from build123d import *

# Parameters (mm, degrees)
SALIENTE_EXTRUIR1_DEPTH      = 7.21
SALIENTE_EXTRUIR2_DEPTH      = 7.21
SALIENTE_EXTRUIR2_DEPTH_BACK = 7.21
CORTAR_EXTRUIR2_DEPTH        = 28.232395202
CORTAR_EXTRUIR2_DEPTH_BACK   = 28.232395202
SALIENTE_EXTRUIR3_START      = -5.2099999
SALIENTE_EXTRUIR3_DEPTH      = 10.4199998
SALIENTE_EXTRUIR3_START_2    = -7.470713012
SALIENTE_EXTRUIR3_2_DEPTH    = 14.941425924
SALIENTE_EXTRUIR3_START_3    = -23.035921246
SALIENTE_EXTRUIR3_3_DEPTH    = 24.035921246


with BuildPart() as part:
    # Croquis1 → Saliente-Extruir1 (new, symmetric)
    with BuildSketch(Plane.XY):
        with BuildLine():
            add(Edge.make_bspline(
                [(-18.945192114, 7.540918896), (-10.215008384, -3.697644103), (-2.846604825, -5.059081104)],
                knots=[0.497667241, 0.497667241, 0.497667241, 0.49955428, 0.49955428, 0.49955428], degree=2, weights=[1, 1, 1]))
            add(Edge.make_bspline(
                [(-2.846604825, -5.059081104), (-0.742366882, -3.9352066), (0.355125, -2.723253227)],
                knots=[0.498812075, 0.498812075, 0.498812075, 0.499412845, 0.499412845, 0.499412845], degree=2, weights=[1, 1, 1]))
            Line((0.355125, -2.723253227), (0.355125, -2.284841781))
            Line((0.355125, -2.284841781), (-1.394875, -2.223730435))
            add(Edge.make_bspline(
                [(-1.394875, -2.223730435), (-0.90753067, -0.123730435), (-1.394875, 1.976269565)],
                knots=[0, 0, 0, 1, 1, 1], degree=2, weights=[1, 3.231801219, 1]))
            Line((-1.394875, 1.976269565), (0.355125, 2.284841781))
            Line((0.355125, 2.284841781), (0.355125, 3.001549529))
            add(Edge.make_bspline(
                [(0.355125, 3.001549529), (-1.44872627, 6.058427314), (-6.994875026, 10.477389992)],
                knots=[0.500820705, 0.500820705, 0.500820705, 0.502013312, 0.502013312, 0.502013312], degree=2, weights=[1, 1, 1]))
            Line((-6.994875026, 10.477389992), (-8.981845695, 12.608155172))
            Line((-8.981845695, 12.608155172), (-23.035921146, 11.871612288))
            Line((-23.035921146, 11.871612288), (-23.035921146, 11.54013782))
            ThreePointArc((-23.035921146, 11.54013782), (-20.949684518, 9.582335705), (-18.945192114, 7.540918896))
        make_face()
    extrude(amount=SALIENTE_EXTRUIR1_DEPTH, both=True)

    # Croquis4 → Saliente-Extruir2 (add, two sides: drawn at the far end of the back side and taken through both)
    with BuildSketch(Plane.XY.offset(-SALIENTE_EXTRUIR2_DEPTH_BACK)):
        Polygon((-1.394875, 1.976269565), (0.355125, 2.284841781), (0.355125, 1.976269565), align=None)
    extrude(amount=SALIENTE_EXTRUIR2_DEPTH + SALIENTE_EXTRUIR2_DEPTH_BACK)

    # Croquis6 → Cortar-Extruir2 (cut, two sides: drawn at the far end of the back side and taken through both)
    with BuildSketch(Plane(origin=(0, 0, 0), x_dir=(0, 0, -1), z_dir=(1, 0, 0)).offset(-CORTAR_EXTRUIR2_DEPTH_BACK)):
        Polygon((7.21, 12.608155172), (7.21, -5.059081104), (5.21, -5.059081104), align=None)
        Polygon((-7.21, 12.608155172), (-7.21, -5.059081104), (-5.21, -5.059081104), align=None)
    extrude(amount=CORTAR_EXTRUIR2_DEPTH + CORTAR_EXTRUIR2_DEPTH_BACK, mode=Mode.SUBTRACT)

    # Saliente-Extruir3: read off the stored shape, not the designer's step
    # Saliente-Extruir3 outline → Saliente-Extruir3 (add)
    with BuildSketch(Plane.XY.offset(SALIENTE_EXTRUIR3_START)):
        with BuildLine():
            add(Edge.make_bspline(
                [(-9.626736117, 12.574357897), (-9.652391468, 12.594799115), (-9.678046818, 12.615240333)],
                knots=[0.502296281, 0.502296281, 0.502296281, 0.502301797, 0.502301797, 0.502301797], degree=2))
            Line((-9.626736117, 12.574357897), (-8.981845695, 12.608155172))
            Line((-8.981845695, 12.608155172), (-6.994875026, 10.477389992))
            add(Edge.make_bspline(
                [(0.355125, 3.001549529), (-1.44872627, 6.058427314), (-6.994875026, 10.477389992)],
                knots=[0.500820705, 0.500820705, 0.500820705, 0.502013312, 0.502013312, 0.502013312], degree=2))
            Line((0.355125, 3.001549529), (0.355125, 14.601784752))
            Line((0.355125, 14.601784752), (-0.813216768, 14.807794929))
            Line((-0.813216768, 14.807794929), (-1.995067613, 14.91119348))
            Line((-1.995067613, 14.91119348), (-3.181432936, 14.91119348))
            Line((-3.181432936, 14.91119348), (-4.363283782, 14.807794929))
            Line((-4.363283782, 14.807794929), (-5.53162555, 14.601784752))
            Line((-5.53162555, 14.601784752), (-6.677566455, 14.294730812))
            Line((-6.677566455, 14.294730812), (-7.792385195, 13.888969974))
            Line((-7.792385195, 13.888969974), (-8.867597325, 13.387590324))
            Line((-8.867597325, 13.387590324), (-9.678046818, 12.615240333))
        make_face()
    extrude(amount=SALIENTE_EXTRUIR3_DEPTH)

    # Saliente-Extruir3 2 outline → Saliente-Extruir3 2 (add)
    with BuildSketch(Plane.XY.offset(SALIENTE_EXTRUIR3_START_2)):
        with BuildLine():
            add(Edge.make_bspline(
                [(-9.626736117, 12.574357897), (-9.652391468, 12.594799115), (-9.678046818, 12.615240333)],
                knots=[0.502296281, 0.502296281, 0.502296281, 0.502301797, 0.502301797, 0.502301797], degree=2))
            Line((-9.626736117, 12.574357897), (-8.981845695, 12.608155172))
            Line((-8.981845695, 12.608155172), (-6.994875026, 10.477389992))
            add(Edge.make_bspline(
                [(0.355125, 3.001549529), (-1.44872627, 6.058427314), (-6.994875026, 10.477389992)],
                knots=[0.500820705, 0.500820705, 0.500820705, 0.502013312, 0.502013312, 0.502013312], degree=2))
            Line((0.355125, 3.001549529), (0.355125, 14.601784752))
            Line((0.355125, 14.601784752), (-0.813216768, 14.807794929))
            Line((-0.813216768, 14.807794929), (-1.995067613, 14.91119348))
            Line((-1.995067613, 14.91119348), (-3.181432936, 14.91119348))
            Line((-3.181432936, 14.91119348), (-4.363283782, 14.807794929))
            Line((-4.363283782, 14.807794929), (-5.53162555, 14.601784752))
            Line((-5.53162555, 14.601784752), (-6.677566455, 14.294730812))
            Line((-6.677566455, 14.294730812), (-7.792385195, 13.888969974))
            Line((-7.792385195, 13.888969974), (-8.867597325, 13.387590324))
            Line((-8.867597325, 13.387590324), (-9.678046818, 12.615240333))
        make_face()
    extrude(amount=SALIENTE_EXTRUIR3_2_DEPTH)

    # Saliente-Extruir3 3 outline → Saliente-Extruir3 3 (cut)
    with BuildSketch(Plane.YZ.offset(SALIENTE_EXTRUIR3_START_3)):
        Polygon((2, 7.470712912), (2, 6.009115492), (14.91119348, 7.470712912), align=None)
        Polygon((14.91119348, -7.470712912), (2, -6.009115492), (2, -7.470713012), align=None)
    extrude(amount=SALIENTE_EXTRUIR3_3_DEPTH, mode=Mode.SUBTRACT)


solid = part.part
Read the model definition and answer for the solid it produces. Units are mm, in the model's axes. Round coordinates to 2 decimals unless told otherwise and drop trailing zeros.
1) The mould has two halves that part along Y. Classify faces 1 (the face through (-1, 1.976, 0)), 2 (the face through (0.355, 8, 0)), 3 (the face through (-0.2, 14.7, -0.1)): released by +Y, released by -Y, zero draft, split by the parting line, or undercut.
2) Flat-ended cylindrical pins translate along their axes: pin 1 (1 mm diameter, centred on y = 1.5, z = -4.5, fed in from -X); pin 2 (8 mm diameter, centred on x = -11, z = -5, fed in from -Y); pin 3 (3 mm diameter, centred on x = -6.5, y = 1.5, fed in from -Z). Find the tip coordinate at first contact, or state that the pin passes through.
3) Straight lines are drawn through the part: L1, parallel to Z at x = -6.75, y = 3; L2, parallel to Y at x = -1.5, z = -3.5; L3, parallel to Y at x = -16.5, z = -6.25. For each, find the intervals that lie inside material, in ascending order.
Resolved:
1. face 1: undercut
1. face 2: zero draft
1. face 3: released by +Y
2. pin 1: stops at x = -14.14
2. pin 2: stops at y = -3.56
2. pin 3: stops at z = -6.12
3. L1: z = -6.12 to 6.12
3. L2: y = -4.26 to 14.87
3. L3: y = 4.56 to 12.21
